```python
from build123d import *

# Parameters (mm, degrees)
F0_W       = 47
F0_H       = 30
F1_DEPTH   = 23
F0_W_2     = 12
F0_H_2     = 3
F2_DEPTH   = 20
F3_W       = 47
F3_H       = 1.2
F4_DEPTH   = 1.2
F5_SIZE    = 0.3
F8_D       = 5.5
F8_ON_F7_D = 5.5
F9_W       = 53
F9_H       = 36
F9_W_2     = 5
F9_H_2     = 10
F9_W_3     = 15
F10_DEPTH  = 3
F11_R      = 3


with BuildPart() as f1:
    # F0 (on Front) → F1 (new body)
    with BuildSketch(Plane.XZ):
        Polygon((-26.5, -18), (26.5, -18), (26.5, -15), (26.5, 18), (-26.5, 18), (-26.5, -15), align=None)
        Rectangle(F0_W, F0_H, mode=Mode.SUBTRACT)
    extrude(amount=F1_DEPTH)

    # F0 (on Front) → F2 (join)
    with BuildSketch(Plane.XZ):
        with Locations((-32.5, -16.5)):
            Rectangle(F0_W_2, F0_H_2)
        with Locations((32.5, -16.5)):
            Rectangle(F0_W_2, F0_H_2)
    extrude(amount=F2_DEPTH)

    # F3 (on face) → F4 (join)
    with BuildSketch(Plane(origin=(0, 0, 0), x_dir=(-1, 0, 0), z_dir=(0, 1, 0))):
        with Locations((0, 14.4)):
            Rectangle(F3_W, F3_H)
        with Locations((0, -14.4)):
            Rectangle(F3_W, F3_H)
    extrude(amount=-F4_DEPTH)

    # F5
    f5_edges = [f1.edges().sort_by_distance(p)[0] for p in [
        (0, 0, -13.8),
        (0, -1.2, -13.8),
        (0, 0, 13.8),
        (0, -1.2, 13.8),
    ]]
    chamfer(f5_edges, length=F5_SIZE)

    # F8 (through all)
    with Locations(Plane.XY.offset(-15)):
        with Locations((-33, -10)):
            Hole(F8_D / 2)

    # F8 on F7 (through all)
    with Locations(Plane.XY.offset(-15)):
        with Locations((33, -10)):
            Hole(F8_ON_F7_D / 2)

    # F9 (on face) → F10 (join)
    with BuildSketch(Plane.XZ.offset(23)):
        Rectangle(F9_W, F9_H)
        with Locations((-17.5, 0)):
            Rectangle(F9_W_2, F9_H_2, mode=Mode.SUBTRACT)
        with Locations((14, 4)):
            Rectangle(F9_W_3, F9_H_2, mode=Mode.SUBTRACT)
    extrude(amount=F10_DEPTH)

    # F11
    f11_edges = [f1.edges().sort_by_distance(p)[0] for p in [
        (-26.5, -10, -15),
        (-26.5, -13, 18),
        (26.5, -13, 18),
        (26.5, -10, -15),
        (26.5, -20, -16.5),
        (-26.5, -20, -16.5),
    ]]
    fillet(f11_edges, radius=F11_R)


solid = f1.part
```
The listing builds one solid part. Answer for the finished solid, in the listing's coordinates (mm). A direction names the side the tool comes from. Round coordinates to 2 decimals unless told otherwise and drop trailing zeros. Write each loop counter-clockwise with the first axis right and the second up, starting at its lowest first coordinate (ties: lowest second). Pieces come first, ordered by that corner, then holes. Notation, with made-up numbers: (68, 73) -> (72, 73) arc R18 ccw to (72, 98) -> close; hole circle Ø4 at (72, -37.75). An arc over 180 degrees is marked (long way). Answer as a JSON object with one key per item and string values. Group by question number.
Q1. Section B-B (x = 33) is taken. Write down the section's boundary in (y, z), plus the area to 3 significant figures.
Q2. Each of these flat-tipped pins is pushed along its axis until it touches: pin 1 Ø0.9 at (y, z) = (-24.5, 3.5) entering from -X; pin 2 Ø0.9 at (x, z) = (-34, -17) entering from -Y; pin 3 Ø5 at (x, y) = (33, -10) entering from -Z; pin 4 Ø15 at (x, z) = (-3.5, 5.5) entering from +Y. Where does it stop, or does it pass through?
Q3. Section D-D (y = -14.25) is taken. Write down the section's boundary in (x, z).
Q4. Determine the mould class of faces 4 (the face through (0, -12, 15)), 5 (the face through (-34, -20, -16)), 6 (the face through (-36, -10, -15)) for opening direction Y: pulls with the +Y half, pulls with the -Y half, needs draft (parallel to the pull), parting line crosses it, or undercut.
Q5. Section C-C (z = -3) is taken. Write down the section's boundary in (x, y).
Q6. Straight lines are drawn through the part: line 1 along Z through (x, y) = (9, -22.5); line 2 along X through (y, z) = (-8.25, -3); line 3 along Y through (x, z) = (33, -15.75). For each, find the intervals that lie inside material, in ascending order.
Q7. Which of the six approach directions +Z, -Z, +X, -X, +Y, -Y give full straight-line access (tool end or side, diameter ignored) to faces 1 (the face through (14, -24, -1)), 2 (the face through (36, -10, -15)), 3 (the face through (0, -12, -15))?
Q8. Section A-A (y = -10) is taken. Write down the section's boundary in (x, z), plus the area to 3 significant figures.
Check values:
{
 "1": {"outline": "(-20, -18) -> (-12.75, -18) -> (-12.75, -15) -> (-20, -15) -> close; (-7.25, -18) -> (0, -18) -> (0, -15) -> (-7.25, -15) -> close", "area": "43.5 mm^2"},
 "2": {"pin 1": "x = -26.5", "pin 2": "y = -20", "pin 3": "through", "pin 4": "y = -23"},
 "3": {"outline": "(-38.5, -18) -> (38.5, -18) -> (38.5, -15) -> (29.5, -15) arc R3 cw to (26.5, -12) -> (26.5, 15) arc R3 ccw to (23.5, 18) -> (-23.5, 18) arc R3 ccw to (-26.5, 15) -> (-26.5, -12) arc R3 cw to (-29.5, -15) -> (-38.5, -15) -> close; hole (-23.5, -15) -> (23.5, -15) -> (23.5, 15) -> (-23.5, 15) -> close"},
 "4": {"face 4": "undercut", "face 5": "pulls with the -Y half", "face 6": "needs draft"},
 "5": {"outline": "(-26.5, -26) -> (-20, -26) -> (-20, -23) -> (-23.5, -23) -> (-23.5, 0) -> (-26.5, 0) -> close; (-15, -26) -> (26.5, -26) -> (26.5, 0) -> (23.5, 0) -> (23.5, -23) -> (-15, -23) -> close"},
 "6": {"line 1": "-18 to -15, 15 to 18", "line 2": "-26.5 to -23.5, 23.5 to 26.5", "line 3": "-20 to -12.75, -7.25 to 0"},
 "7": {"face 1": "+Y, -Y", "face 2": "+Z, +X, +Y, -Y", "face 3": "none"},
 "8": {"outline": "(-38.5, -18) -> (-35.75, -18) -> (-35.75, -15) -> (-38.5, -15) -> close; (-30.25, -18) -> (30.25, -18) -> (30.25, -15) -> (29.5, -15) arc R3 cw to (26.5, -12) -> (26.5, 15) arc R3 ccw to (23.5, 18) -> (-23.5, 18) arc R3 ccw to (-26.5, 15) -> (-26.5, -12) arc R3 cw to (-29.5, -15) -> (-30.25, -15) -> close; (35.75, -18) -> (38.5, -18) -> (38.5, -15) -> (35.75, -15) -> close; hole (-23.5, -15) -> (23.5, -15) -> (23.5, 15) -> (-23.5, 15) -> close", "area": "537 mm^2"}
}
